from build123d import *

# Parameters (mm, degrees)
F0_W     = 812.8
F0_H     = 1016
F1_DEPTH = 9.525
F3_D     = 47.625
F4_D     = 19.05
F5_D     = 22.86


with BuildPart() as f1:
    # F0 (on Front) → F1 (new body)
    with BuildSketch(Plane.XZ):
        with Locations((-368.4664566755, 476.7986876816)):
            Rectangle(F0_W, F0_H)
    extrude(amount=F1_DEPTH)

    # F3 (through all)
    with Locations(Plane(origin=(0, 0, 0), x_dir=(1, 0, 0), z_dir=(0, 1, 0))):
        with Locations((-722.4662566755, -940.3486876816), (-722.4662566755, -13.2486876816)):
            Hole(F3_D / 2)

    # F4 (through all)
    with Locations(Plane(origin=(0, 0, 0), x_dir=(1, 0, 0), z_dir=(0, 1, 0))):
        with Locations((-685.9664566755, -476.7986876816)):
            Hole(F4_D / 2)

    # F5 (through all)
    with Locations(Plane(origin=(0, 0, 0), x_dir=(1, 0, 0), z_dir=(0, 1, 0))):
        with Locations((-641.5164566755, -784.7736876816), (-298.6164566755, -476.7986876816), (12.5335433245, -784.7736876816), (12.5335433245, -168.8236876816), (-641.5164566755, -168.8236876816)):
            Hole(F5_D / 2)


solid = f1.part
Could you check a few things on this model? Use its own coordinates, in mm. Coordinates: 2 decimals unless noted, no trailing zeros. One line per item, written item: value. Start each with the question number.
1) We'd pull the mould along Z, two halves only. Please class faces 1 (the cylindrical face through (15.011, -4.829, 179.982)), 2 (the flat face through (-374, 0, 484)): +Z half, -Z half, draft (parallel to the pull), parting line (faces both ways), or undercut.
2) I'm going to push a flat-ended pin straight in: pin 1 (10 mm diameter, centred on x = -349.5, z = 333, fed in from +Y). Where does the tip first touch, or does it pass through?
3) If I drill on L1, parallel to X at y = -3.25, z = 479; L2, parallel to X at y = -2, z = 943.5; L3, parallel to Z at x = -735, y = -6.5, over which ranges is the centre line in solid material (lowest first)? Write a range as [from, to].
Answer list:
1. face 1: undercut
1. face 2: draft
2. pin 1: stops at y = 0
3. L1: x = [-774.87, -695.23], [-676.7, -309.83], [-287.4, 37.93]
3. L2: x = [-774.87, -746.07], [-698.86, 37.93]
3. L3: z = [-31.2, -7], [33.5, 920.1], [960.6, 984.8]
